Geometry: see drawing. Coordinates: mm, zero at the bounding-box minimum. A direction names the side the tool comes from. Give positions to 0.01 mm unless a question says otherwise; leave off trailing zeros. Order: outer loops, then holes, each group sorted by start corner. A loop starts at its lowest first (then second) coordinate and runs counter-clockwise, first axis right, second up. Notation, with made-up numbers: (47, 58.25) - (100, 58.25) arc R31 ccw to (100, 93.25) - close; hole circle Ø5 at (74.5, -6). An arc over 180 degrees is marked (long way). Write each question's results on one line, items separated by ' | '. Start each with the question number.
Item 1: Mould query, pull axis X, two halves, no side actions, for the marked faces 5, 6, 7 and 8. Classes: released by +X, released by -X, zero draft, split by the parting line, or undercut.
Item 2: Section B-B on y = 17.4. State how many separate pieces and enclosed holes the cut face has.
Item 3: Section A-A on z = 6.35. Output: boundary loops of the cut face in (x, y).
Item 4: Set-up query: the marked faces 1, 2, 3 and 4. Return all of +Z, -Z, +X, -X, +Y, -Y with unobstructed straight access to the full face (end or side cutting, diameter ignored); none if empty.
Item 5: Section C-C on x = 11.5. Output: boundary loops of the cut face in (y, z) (1 decimal).
Item 6: Line query: line 1 along X through (y, z) = (4, 69.85); line 2 along X through (y, z) = (14, 25.5) (1 decimal); line 3 along Y through (x, z) = (56.75, 53.1). Output: solid intervals per line, ascending.
Item 7: Contact query for flat-ended pins moving along their axis: pin 1 Ø2 at (x, y) = (53.5, 18.5) entering from -Z; pin 2 Ø5 at (x, z) = (19.5, 51.5) entering from -Y; pin 3 Ø5 at (y, z) = (17.4, 23.1) entering from -X; pin 4 Ø2.5 at (y, z) = (17.4, 23.1) entering from -X. Output: stop coordinate, or through.
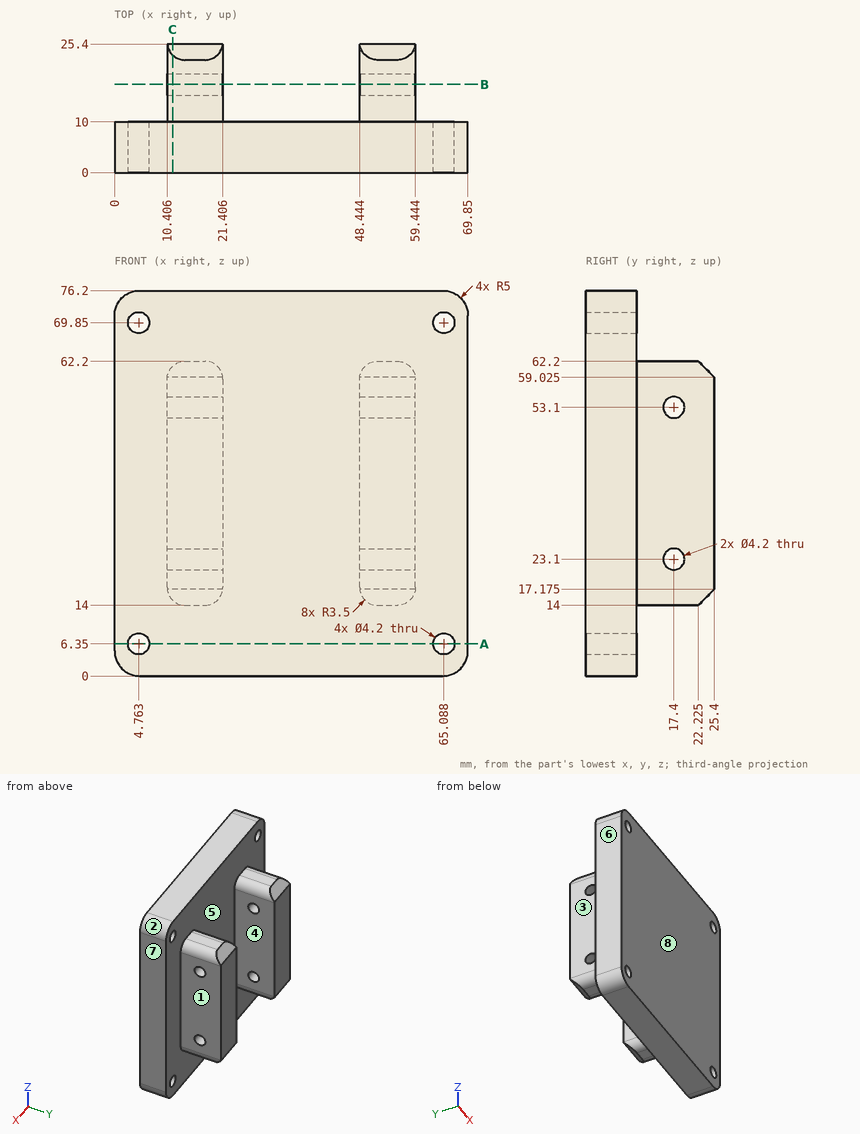
Evaluation:
1) face 5: undercut | face 6: released by -X | face 7: released by +X | face 8: zero draft
2) separate pieces: 6 | enclosed holes: 0
3) outline: (0, 0) - (2.66, 0) - (2.66, 10) - (0, 10) - close; (6.86, 0) - (62.99, 0) - (62.99, 10) - (6.86, 10) - close; (67.19, 0) - (69.85, 0) - (69.85, 10) - (67.19, 10) - close
4) face 1: +Z, -Z, +X, +Y | face 2: +Z, +X, +Y, -Y | face 3: +Z, -Z, -X, +Y | face 4: +Z, -Z, +Y
5) outline: (0, 0) - (10, 0) - (10, 15) - (23.2, 15) - (25.4, 17.2) - (25.4, 59) - (23.2, 61.2) - (10, 61.2) - (10, 76.2) - (0, 76.2) - close; hole circle Ø4.2 at (17.4, 23.1); hole circle Ø4.2 at (17.4, 53.1)
6) line 1: x = 0 to 2.66, 6.86 to 62.99, 67.19 to 69.85 | line 2: x = 10.4 to 21.4, 48.4 to 59.4 | line 3: y = 0 to 15.3, 19.5 to 25.4
7) pin 1: stops at z = 14 | pin 2: stops at y = 0 | pin 3: stops at x = 10.41 | pin 4: passes through
